Work out the finished part from the listing and answer in its coordinate system (mm). A direction names the side the tool comes from. Round coordinates to 2 decimals unless told otherwise and drop trailing zeros. Write each loop counter-clockwise with the first axis right and the second up, starting at its lowest first coordinate (ties: lowest second). Pieces come first, ordered by that corner, then holes.
1. Find section B-B (x = 3). Write down the section's boundary in (y, z).
2. Find section C-C (x = -10). Count the separate pieces of the cut face and the enclosed holes in it, and give its area (3 significant figures).
3. Flat-ended cylindrical pins translate along their axes: pin 1 Ø3 at (x, z) = (-3.5, 9) entering from +Y; pin 2 Ø0.5 at (x, y) = (10, 1.5) entering from -Z; pin 3 Ø0.5 at (x, y) = (-10.5, 1.5) entering from +Z; pin 4 Ø1.3 at (x, z) = (9.6, -18.65) entering from +Y. Find the tip coordinate at first contact, or state that the pin passes through.
4. Find section A-A (z = -0.5). Write down the section's boundary in (x, y).
5. Determine the mould class of faces 1 (the face through (7.847, 2.014, 16.868)), 2 (the face through (0.09, 0.49, -20.64)), 3 (the face through (11, 2, -19)) for opening direction Z: pulls with the +Z half, pulls with the -Z half, needs draft (parallel to the pull), parting line crosses it, or undercut.
6. Straight lines are drawn through the part: probe 1 along Z at (x, y) = (2.75, 2.6); probe 2 along Z at (x, y) = (9.6, 2.6); probe 3 along X at (y, z) = (2.75, 18.65). For each, find the intervals that lie inside material, in ascending order.
7. A tool of negligible diameter and unlimited length cuts with its end or side. For faces 4 (the face through (7.7, 1.5, -19.2)), 5 (the face through (0, 2, 20.15)), 6 (the face through (-11, 2, -19)), 7 (the face through (8, 2, 19)), 8 (the face through (10.959, 2.507, -19.947)), from which of +Z, -Z, +X, -X, +Y, -Y can it reach the whole face along a straight path? Write none if from no direction.
```python
from build123d import *

# Parameters (mm, degrees)
SKETCH_1_W               = 24.2
SKETCH_1_H               = 42.3
EXTRUDE_1_DEPTH          = 3
FILLET_1_R               = 4
CUT_EXTRUDE_1_DEPTH      = 2
EXTRUDE_START            = 2
EXTRUDE_2_DEPTH          = 2
FILLET_2_R               = 2.5
CUT_EXTRUDE_2_DEPTH      = 25.550611138
CUT_EXTRUDE_2_DEPTH_BACK = 25.550611138
SKETCH_4_R               = 1.1
CUT_EXTRUDE_3_DEPTH      = 2
FILLET_3_R               = 1.5
CHAMFER_1_SIZE           = 1


with BuildPart() as part:
    # 草图1 → 凸台-拉伸1 (new body)
    with BuildSketch(Plane(origin=(0, 0, 0), x_dir=(1, 0, 0), z_dir=(0, 1, 0))):
        Rectangle(SKETCH_1_W, SKETCH_1_H)
    extrude(amount=EXTRUDE_1_DEPTH)

    # 圆角1
    fillet_1_edges = [part.edges().sort_by_distance(p)[0] for p in [
        (12.1, 1.5, 21.15),
        (-12.1, 1.5, 21.15),
        (-12.1, 1.5, -21.15),
        (12.1, 1.5, -21.15),
    ]]
    fillet(fillet_1_edges, radius=FILLET_1_R)

    # 草图2 → 切除-拉伸1 (cut)
    with BuildSketch(Plane(origin=(0, 3, 0), x_dir=(1, 0, 0), z_dir=(0, 1, 0))):
        with BuildLine():
            Line((8.1, 20.15), (-8.1, 20.15))
            ThreePointArc((-8.1, 20.15), (-10.221320344, 19.271320344), (-11.1, 17.15))
            Line((-11.1, 17.15), (-11.1, -17.15))
            ThreePointArc((-11.1, -17.15), (-10.221320344, -19.271320344), (-8.1, -20.15))
            Line((-8.1, -20.15), (8.1, -20.15))
            ThreePointArc((8.1, -20.15), (10.221320344, -19.271320344), (11.1, -17.15))
            Line((11.1, -17.15), (11.1, 17.15))
            ThreePointArc((11.1, 17.15), (10.221320344, 19.271320344), (8.1, 20.15))
        make_face()
    extrude(amount=-CUT_EXTRUDE_1_DEPTH, mode=Mode.SUBTRACT)

    # 草图3 → 凸台-拉伸2 (add)
    with BuildSketch(Plane(origin=(0, 1, 0), x_dir=(1, 0, 0), z_dir=(0, 1, 0)).offset(EXTRUDE_START)):
        with BuildLine():
            Line((-9.6, 16.15), (-11.1, 16.15))
            Line((-11.1, 16.15), (-11.1, 17.15))
            ThreePointArc((-11.1, 17.15), (-10.221320344, 19.271320344), (-8.1, 20.15))
            Line((-8.1, 20.15), (-7.1, 20.15))
            Line((-7.1, 20.15), (-7.1, 18.65))
            ThreePointArc((-7.1, 18.65), (-7.832233047, 16.882233047), (-9.6, 16.15))
        make_face()
        with BuildLine():
            Line((7.1, 18.65), (7.1, 20.15))
            Line((7.1, 20.15), (8.1, 20.15))
            ThreePointArc((8.1, 20.15), (10.221320344, 19.271320344), (11.1, 17.15))
            Line((11.1, 17.15), (11.1, 16.15))
            Line((11.1, 16.15), (9.6, 16.15))
            ThreePointArc((9.6, 16.15), (7.832233047, 16.882233047), (7.1, 18.65))
        make_face()
        with BuildLine():
            Line((-8.1, -20.15), (-7.1, -20.15))
            Line((-7.1, -20.15), (-7.1, -18.65))
            ThreePointArc((-7.1, -18.65), (-7.832233047, -16.882233047), (-9.6, -16.15))
            Line((-9.6, -16.15), (-11.1, -16.15))
            Line((-11.1, -16.15), (-11.1, -17.15))
            ThreePointArc((-11.1, -17.15), (-10.221320344, -19.271320344), (-8.1, -20.15))
        make_face()
        with BuildLine():
            Line((11.1, -17.15), (11.1, -16.15))
            Line((11.1, -16.15), (9.6, -16.15))
            ThreePointArc((9.6, -16.15), (7.832233047, -16.882233047), (7.1, -18.65))
            Line((7.1, -18.65), (7.1, -20.15))
            Line((7.1, -20.15), (8.1, -20.15))
            ThreePointArc((8.1, -20.15), (10.221320344, -19.271320344), (11.1, -17.15))
        make_face()
    extrude(amount=-EXTRUDE_2_DEPTH)

    # 圆角2
    fillet_2_edges = [part.edges().sort_by_distance(p)[0] for p in [
        (7.1, 2, 20.15),
        (11.1, 2, 16.15),
        (11.1, 2, -16.15),
        (7.1, 2, -20.15),
        (-7.1, 2, -20.15),
        (-11.1, 2, 16.15),
        (-7.1, 2, 20.15),
        (-11.1, 2, -16.15),
    ]]
    fillet(fillet_2_edges, radius=FILLET_2_R)

    # 草图4 → 切除-拉伸2 (cut, two sides: drawn at the far end of the back side and taken through both)
    with BuildSketch(Plane.XZ.offset(-CUT_EXTRUDE_2_DEPTH_BACK)):
        with Locations(Location((-9.6, 18.65, 0), (0, 0, 270))):
            Circle(SKETCH_4_R)
        with Locations(Location((9.6, 18.65, 0), (0, 0, 270))):
            Circle(SKETCH_4_R)
        with Locations(Location((9.6, -18.65, 0), (0, 0, 270))):
            Circle(SKETCH_4_R)
        with Locations(Location((-9.6, -18.65, 0), (0, 0, 270))):
            Circle(SKETCH_4_R)
    extrude(amount=CUT_EXTRUDE_2_DEPTH + CUT_EXTRUDE_2_DEPTH_BACK, mode=Mode.SUBTRACT)

    # 草图5 → 切除-拉伸3 (cut)
    with BuildSketch(Plane.XZ):
        with BuildLine():
            Line((-9.6, 16.75), (-12.1, 16.75))
            Line((-12.1, 16.75), (-12.1, 21.15))
            Line((-12.1, 21.15), (-7.7, 21.15))
            Line((-7.7, 21.15), (-7.7, 18.65))
            ThreePointArc((-7.7, 18.65), (-8.256497116, 17.306497116), (-9.6, 16.75))
        make_face()
        with BuildLine():
            Line((9.6, 16.75), (12.1, 16.75))
            Line((12.1, 16.75), (12.1, 21.15))
            Line((12.1, 21.15), (7.7, 21.15))
            Line((7.7, 21.15), (7.7, 18.65))
            ThreePointArc((7.7, 18.65), (8.256497116, 17.306497116), (9.6, 16.75))
        make_face()
        with BuildLine():
            Line((9.6, -16.75), (12.1, -16.75))
            Line((12.1, -16.75), (12.1, -21.15))
            Line((12.1, -21.15), (7.7, -21.15))
            Line((7.7, -21.15), (7.7, -18.65))
            ThreePointArc((7.7, -18.65), (8.256497116, -17.306497116), (9.6, -16.75))
        make_face()
        with BuildLine():
            Line((-9.6, -16.75), (-12.1, -16.75))
            Line((-12.1, -16.75), (-12.1, -21.15))
            Line((-12.1, -21.15), (-7.7, -21.15))
            Line((-7.7, -21.15), (-7.7, -18.65))
            ThreePointArc((-7.7, -18.65), (-8.256497116, -17.306497116), (-9.6, -16.75))
        make_face()
    extrude(amount=-CUT_EXTRUDE_3_DEPTH, mode=Mode.SUBTRACT)

    # 圆角3
    fillet_3_edges = [part.edges().sort_by_distance(p)[0] for p in [
        (-7.7, 1, -21.15),
        (-12.1, 1, -16.75),
        (12.1, 1, -16.75),
        (7.7, 1, -21.15),
        (7.7, 1, 21.15),
        (12.1, 1, 16.75),
        (-12.1, 1, 16.75),
        (-7.7, 1, 21.15),
    ]]
    fillet(fillet_3_edges, radius=FILLET_3_R)

    # 倒角1
    chamfer_1_edges = [part.edges().sort_by_distance(p)[0] for p in [
        (-8.256497116, 0, -17.306497116),
        (-10.1, 0, -16.75),
        (8.256497116, 0, -17.306497116),
        (7.7, 0, -19.15),
        (8.256497116, 0, 17.306497116),
        (10.1, 0, 16.75),
        (-8.256497116, 0, 17.306497116),
        (-7.7, 0, 19.15),
        (-12.1, 0, 0),
        (-7.7, 0, -19.15),
        (0, 0, -21.15),
        (10.1, 0, -16.75),
        (12.1, 0, 0),
        (7.7, 0, 19.15),
        (0, 0, 21.15),
        (-10.1, 0, 16.75),
        (-11.660660172, 0, 16.310660172),
        (-7.260660172, 0, -20.710660172),
        (7.260660172, 0, -20.710660172),
        (11.660660172, 0, -16.310660172),
        (11.660660172, 0, 16.310660172),
        (7.260660172, 0, 20.710660172),
        (-7.260660172, 0, 20.710660172),
        (-11.660660172, 0, -16.310660172),
    ]]
    chamfer(chamfer_1_edges, length=CHAMFER_1_SIZE)


solid = part.part
```
Worked answers:
1. outline: (0, -20.15) - (1, -21.15) - (3, -21.15) - (3, -20.15) - (1, -20.15) - (1, 20.15) - (3, 20.15) - (3, 21.15) - (1, 21.15) - (0, 20.15) - close
2. separate pieces: 3
2. enclosed holes: 0
2. area: 40.0 mm2
3. pin 1: stops at y = 1
3. pin 2: stops at z = -16.75
3. pin 3: stops at z = 16.75
3. pin 4: passes through
4. outline: (-12.1, 1) - (-11.1, 0) - (11.1, 0) - (12.1, 1) - (12.1, 3) - (11.1, 3) - (11.1, 1) - (-11.1, 1) - (-11.1, 3) - (-12.1, 3) - close
5. face 1: undercut
5. face 2: pulls with the -Z half
5. face 3: needs draft
6. probe 1: z = -21.15 to -20.15, 20.15 to 21.15
6. probe 2: z = -20.86 to -19.75, -17.55 to -16.04, 16.04 to 17.55, 19.75 to 20.86
6. probe 3: x = -11.81 to -10.7, -8.5 to -6.99, 6.99 to 8.5, 10.7 to 11.81
7. face 4: -Z, +X, -Y
7. face 5: +Y
7. face 6: -Z, -X, -Y
7. face 7: +Z, +X, -Y
7. face 8: -Z, +X, +Y, -Y
